```python
from build123d import *

# Parameters (mm, degrees)
CROQUIS1_R              = 70
SALIENTE_EXTRUIR1_DEPTH = 5
CROQUIS2_R              = 30
SALIENTE_EXTRUIR2_DEPTH = 60
CROQUIS5_R              = 5.25
CORTAR_EXTRUIR5_DEPTH   = 10
CROQUIS7_R              = 25
CORTAR_EXTRUIR6_DEPTH   = 35


with BuildPart() as part:
    # Croquis1 → Saliente-Extruir1 (new body)
    with BuildSketch(Plane(origin=(0, 0, 0), x_dir=(1, 0, 0), z_dir=(0, 1, 0))):
        with Locations(Location((0, 0, 0), (0, 0, 270))):
            Circle(CROQUIS1_R)
    extrude(amount=SALIENTE_EXTRUIR1_DEPTH)

    # Croquis2 → Saliente-Extruir2 (add)
    with BuildSketch(Plane(origin=(0, 5, 0), x_dir=(1, 0, 0), z_dir=(0, 1, 0))):
        with Locations(Location((0, 0, 0), (0, 0, 270))):
            Circle(CROQUIS2_R)
    extrude(amount=SALIENTE_EXTRUIR2_DEPTH)

    # Croquis5 → Cortar-Extruir5 (cut)
    with BuildSketch(Plane.XZ):
        with Locations(Location((0, 0, 0), (0, 0, 270))):
            Circle(CROQUIS5_R)
    extrude(amount=-CORTAR_EXTRUIR5_DEPTH, mode=Mode.SUBTRACT)

    # Croquis7 → Cortar-Extruir6 (cut)
    with BuildSketch(Plane(origin=(0, 65, 0), x_dir=(1, 0, 0), z_dir=(0, 1, 0))):
        with Locations(Location((0, 0, 0), (0, 0, 270))):
            Circle(CROQUIS7_R)
    extrude(amount=-CORTAR_EXTRUIR6_DEPTH, mode=Mode.SUBTRACT)


solid = part.part
```
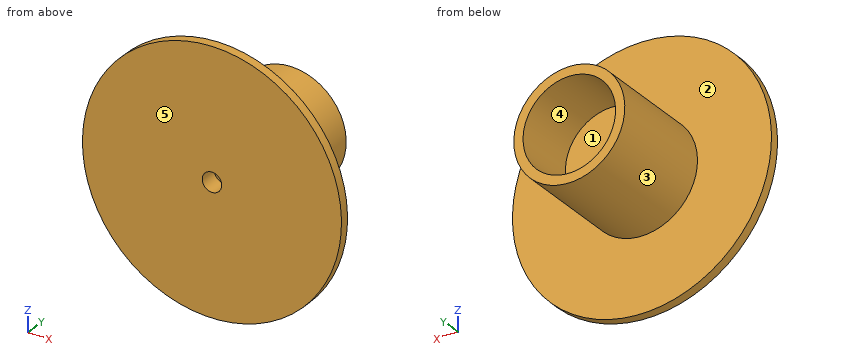
Work out the finished part from the listing and answer in its coordinate system (mm). Face numbers are marked on the shaded views. A direction names the side the tool comes from. Round coordinates to 2 decimals unless told otherwise and drop trailing zeros. Write each loop counter-clockwise with the first axis right and the second up, starting at its lowest first coordinate (ties: lowest second). Pieces come first, ordered by that corner, then holes.
1) A cutting plane is placed at C-C on y = 52. Determine the outline of the cut face in (x, z).
2) Consider probe 1 along X at (y, z) = (4, 0); probe 2 along X at (y, z) = (45, 0); probe 3 along Y at (x, z) = (32, 21). Determine where each line is inside the solid, lowest interval first.
3) Determine the mould class of the marked faces 1, 2 and 3 for opening direction Z: pulls with the +Z half, pulls with the -Z half, needs draft (parallel to the pull), parting line crosses it, or undercut.
4) A cutting plane is placed at A-A on x = 0. Determine the outline of the cut face in (y, z).
5) A cutting plane is placed at D-D on y = 17. Determine the outline of the cut face in (x, z), and give its area (3 significant figures).
6) Flat-ended cylindrical pins translate along their axes: P1, Ø3, axis at x = -2, z = 1, coming from the -Y side; P2, Ø9.5, axis at x = 0, z = 0, coming from the +Y side; P3, Ø1.5, axis at x = -15.5, y = 9, coming from the -Z side. Find the tip coordinate at first contact, or state that the pin passes through.
7) Which of the six approach directions +Z, -Z, +X, -X, +Y, -Y give full straight-line access (tool end or side, diameter ignored) to the marked faces 4 and 5?
8) A cutting plane is placed at B-B on z = 0. Determine the outline of the cut face in (x, y), and give its area (4 significant figures).
Entries:
1. outline: circle Ø60 at (0, 0); hole circle Ø50 at (0, 0)
2. probe 1: x = -70 to -5.25, 5.25 to 70
2. probe 2: x = -30 to -25, 25 to 30
2. probe 3: y = 0 to 5
3. face 1: undercut
3. face 2: needs draft
3. face 3: parting line crosses it
4. outline: (0, -70) - (5, -70) - (5, -30) - (65, -30) - (65, -25) - (30, -25) - (30, 25) - (65, 25) - (65, 30) - (5, 30) - (5, 70) - (0, 70) - (0, 5.25) - (10, 5.25) - (10, -5.25) - (0, -5.25) - close
5. outline: circle Ø60 at (0, 0)
5. area: 2,830 mm2
6. P1: stops at y = 10
6. P2: stops at y = 30
6. P3: stops at z = -26.12
7. face 4: +Y
7. face 5: +Z, -Z, +X, -X, -Y
8. outline: (-70, 0) - (-5.25, 0) - (-5.25, 10) - (5.25, 10) - (5.25, 0) - (70, 0) - (70, 5) - (30, 5) - (30, 65) - (25, 65) - (25, 30) - (-25, 30) - (-25, 65) - (-30, 65) - (-30, 5) - (-70, 5) - close
8. area: 2,445 mm2
